Geometry check sheet. Reference: the model listing, model coordinates, mm. A direction names the side the tool comes from. Round coordinates to 2 decimals unless told otherwise and drop trailing zeros. Loops run counter-clockwise (first coordinate to the right, second up) from the corner with the lowest first, then second, coordinate; pieces in that order, holes last. Notation, with made-up numbers: M -37,9.25 L 3,9.25 A17 cw 3,31.25 Z; hole C -12,33 d10. An arc over 180 degrees is marked long. Use one line per item in the form item = value. Start each with the question number.
1. Set-up check for faces 1 (the flat face through (-109, 53, -2)), 2 (the flat face through (-2, 43, -8)), 3 (the conical face through (-171.003, 19.14, -1.875)): record each of +Z, -Z, +X, -X, +Y, -Y from which the full face is reachable in a straight line by a thin tool's end or side.
2. Go/stop test with flat-tipped pins: pin 1 (5 mm diameter, centred on x = -13.38, y = 72.07, fed in from +Z); pin 2 (5 mm diameter, centred on x = -81.5, y = 39.5, fed in from -Z); pin 3 (4 mm diameter, centred on x = -13.38, y = 19.07, fed in from +Z). Record where each tip stops, or that it passes through.
3. Cross-section at D-D (x = -69). Record the boundary of the cut face in (y, z), then the cut area to 3 significant figures.
4. Material ranges on line 1 (Y direction, x = -7.5, z = -4.25); line 2 (X direction, y = 38.5, z = -6); line 3 (Y direction, x = -13, z = -2.5), recorded low to high.
5. Cross-section at B-B (x = -124). Record the boundary of the cut face in (y, z).
6. Draft check along X on faces 4 (the flat face through (-89, 84, -7)), 5 (the flat face through (-91, 43, -4)). Enter one of: pulls with the +X half, pulls with the -X half, needs draft (parallel to the pull), parting line crosses it, or undercut.
7. Cross-section at C-C (z = -7.25). Record the boundary of the cut face in (x, y).
8. Cross-section at A-A (y = 50). Record the boundary of the cut face in (x, z).
```python
from build123d import *

# Parameters (mm, degrees)
F1_DEPTH = 11.5
F0_R     = 1.5
F2_DEPTH = 4
F3_SIZE  = 2
F4_W     = 27.3790522566
F4_H     = 13
F5_DEPTH = 25


# Not quite as in the source:
# - a feature names something its author has since deleted; it is built from what else it names


with BuildPart() as f1:
    # F0 (on Top) → F1 (new body)
    with BuildSketch(Plane.XY):
        Polygon((-180.3790522566, 0), (0, 0), (0, 42), (0, 84), (-180.3790522566, 84), align=None)
        Polygon((-2, 82), (-2, 42), (-2, 2), (-35, 2), (-178.3790522566, 2), (-178.3790522566, 82), (-35, 82), align=None, mode=Mode.SUBTRACT)
    extrude(amount=-F1_DEPTH)

    # F0 (on Top) → F2 (join)
    with BuildSketch(Plane.XY):
        Polygon((-35, 76.0685783849), (-35, 82), (-178.3790522566, 82), (-178.3790522566, 2), (-35, 2), (-35, 15.0685783849), (-63, 15.0685783849), (-173.3790522566, 15.0685783849), (-173.3790522566, 76.0685783849), align=None)
        with BuildLine():
            Line((-35, 63), (-35, 76.0685783849))
            Line((-35, 76.0685783849), (-173.3790522566, 76.0685783849))
            Line((-173.3790522566, 76.0685783849), (-173.3790522566, 15.0685783849))
            Line((-173.3790522566, 15.0685783849), (-63, 15.0685783849))
            Line((-63, 15.0685783849), (-63, 21.5))
            Line((-63, 21.5), (-163, 21.5))
            Line((-163, 21.5), (-163, 62.5))
            Line((-163, 62.5), (-63, 62.5))
            Line((-63, 62.5), (-63, 42))
            Line((-63, 42), (-56, 42))
            ThreePointArc((-56, 42), (-51, 47), (-46, 42))
            Line((-46, 42), (-40, 42))
            ThreePointArc((-40, 42), (-38.5355339059, 45.5355339059), (-35, 47))
            Line((-35, 47), (-35, 53))
            ThreePointArc((-35, 53), (-40, 58), (-35, 63))
        make_face()
        with Locations((-169.3790522566, 19.0685783849)):
            Circle(F0_R, mode=Mode.SUBTRACT)
        with Locations((-169.3790522566, 72.0685783849)):
            Circle(F0_R, mode=Mode.SUBTRACT)
        with BuildLine():
            Line((-14, 42), (-9.3790522566, 42))
            Line((-9.3790522566, 42), (-9.3790522566, 76.0685783849))
            Line((-9.3790522566, 76.0685783849), (-35, 76.0685783849))
            Line((-35, 76.0685783849), (-35, 63))
            ThreePointArc((-35, 63), (-31.4644660941, 61.5355339059), (-30, 58))
            ThreePointArc((-30, 58), (-31.4644660941, 54.4644660941), (-35, 53))
            Line((-35, 53), (-35, 47))
            ThreePointArc((-35, 47), (-31.4644660941, 45.5355339059), (-30, 42))
            Line((-30, 42), (-24, 42))
            ThreePointArc((-24, 42), (-19, 47), (-14, 42))
        make_face()
        with Locations((-13.3790522566, 72.0685783849)):
            Circle(F0_R, mode=Mode.SUBTRACT)
        Polygon((-9.3790522566, 42), (-2, 42), (-2, 82), (-35, 82), (-35, 76.0685783849), (-9.3790522566, 76.0685783849), align=None)
        Polygon((-2, 2), (-2, 42), (-9.3790522566, 42), (-9.3790522566, 15.0685783849), (-35, 15.0685783849), (-35, 2), align=None)
        with BuildLine():
            Line((-9.3790522566, 15.0685783849), (-9.3790522566, 42))
            Line((-9.3790522566, 42), (-14, 42))
            ThreePointArc((-14, 42), (-19, 37), (-24, 42))
            Line((-24, 42), (-30, 42))
            ThreePointArc((-30, 42), (-31.4644660941, 38.4644660941), (-35, 37))
            Line((-35, 37), (-35, 31))
            ThreePointArc((-35, 31), (-31.4644660941, 29.5355339059), (-30, 26))
            ThreePointArc((-30, 26), (-31.4644660941, 22.4644660941), (-35, 21))
            Line((-35, 21), (-35, 15.0685783849))
            Line((-35, 15.0685783849), (-9.3790522566, 15.0685783849))
        make_face()
        with Locations((-13.3790522566, 19.0685783849)):
            Circle(F0_R, mode=Mode.SUBTRACT)
        with BuildLine():
            Line((-63, 15.0685783849), (-35, 15.0685783849))
            Line((-35, 15.0685783849), (-35, 21))
            ThreePointArc((-35, 21), (-40, 26), (-35, 31))
            Line((-35, 31), (-35, 37))
            ThreePointArc((-35, 37), (-38.5355339059, 38.4644660941), (-40, 42))
            Line((-40, 42), (-46, 42))
            ThreePointArc((-46, 42), (-51, 37), (-56, 42))
            Line((-56, 42), (-63, 42))
            Line((-63, 42), (-63, 21.5))
            Line((-63, 21.5), (-63, 15.0685783849))
        make_face()
        with BuildLine():
            Line((-46, 42), (-56, 42))
            ThreePointArc((-56, 42), (-51, 37), (-46, 42))
        make_face()
        with BuildLine():
            ThreePointArc((-46, 42), (-51, 47), (-56, 42))
            Line((-56, 42), (-46, 42))
        make_face()
        with BuildLine():
            ThreePointArc((-35, 37), (-31.4644660941, 38.4644660941), (-30, 42))
            Line((-30, 42), (-35, 42))
            Line((-35, 42), (-35, 37))
        make_face()
        with BuildLine():
            Line((-35, 42), (-30, 42))
            ThreePointArc((-30, 42), (-31.4644660941, 45.5355339059), (-35, 47))
            Line((-35, 47), (-35, 42))
        make_face()
        with BuildLine():
            ThreePointArc((-40, 42), (-38.5355339059, 38.4644660941), (-35, 37))
            Line((-35, 37), (-35, 42))
            Line((-35, 42), (-40, 42))
        make_face()
        with BuildLine():
            Line((-35, 42), (-35, 47))
            ThreePointArc((-35, 47), (-38.5355339059, 45.5355339059), (-40, 42))
            Line((-40, 42), (-35, 42))
        make_face()
        with BuildLine():
            ThreePointArc((-24, 42), (-19, 37), (-14, 42))
            Line((-14, 42), (-24, 42))
        make_face()
        with BuildLine():
            Line((-24, 42), (-14, 42))
            ThreePointArc((-14, 42), (-19, 47), (-24, 42))
        make_face()
        with BuildLine():
            ThreePointArc((-30, 58), (-31.4644660941, 61.5355339059), (-35, 63))
            Line((-35, 63), (-35, 58))
            Line((-35, 58), (-35, 53))
            ThreePointArc((-35, 53), (-31.4644660941, 54.4644660941), (-30, 58))
        make_face()
        with BuildLine():
            Line((-35, 58), (-35, 63))
            ThreePointArc((-35, 63), (-40, 58), (-35, 53))
            Line((-35, 53), (-35, 58))
        make_face()
        with BuildLine():
            Line((-35, 26), (-35, 21))
            ThreePointArc((-35, 21), (-31.4644660941, 22.4644660941), (-30, 26))
            ThreePointArc((-30, 26), (-31.4644660941, 29.5355339059), (-35, 31))
            Line((-35, 31), (-35, 26))
        make_face()
        with BuildLine():
            ThreePointArc((-35, 31), (-40, 26), (-35, 21))
            Line((-35, 21), (-35, 26))
            Line((-35, 26), (-35, 31))
        make_face()
        Polygon((-163, 21.5), (-63, 21.5), (-63, 42), (-63, 62.5), (-163, 62.5), align=None)
    extrude(amount=-F2_DEPTH)

    # F3
    f3_edges = [f1.edges().sort_by_distance(p)[0] for p in [
        (-90.189526, 84, 0),
        (0, 42, 0),
        (-90.189526, 0, 0),
        (-180.379052, 42, 0),
        (-170.879052, 19.068578, 0),
        (-14.879052, 72.068578, 0),
        (-14.879052, 19.068578, 0),
        (-170.879052, 72.068578, 0),
    ]]
    chamfer(f3_edges, length=F3_SIZE)

    # F4 (on face) → F5 (cut)
    with BuildSketch(Plane.XY):
        with Locations((-122.6895261283, 53.5)):
            Rectangle(F4_W, F4_H)
    extrude(amount=-F5_DEPTH, mode=Mode.SUBTRACT)


solid = f1.part
```
Reported:
q1.face_1 = +Z, -Z
q1.face_2 = -Z
q1.face_3 = +Z
q2.pin_1 = -1
q2.pin_2 = -4
q2.pin_3 = -1.5
q3.outline = M 0,-11.5 L 2,-11.5 L 2,-4 L 82,-4 L 82,-11.5 L 84,-11.5 L 84,-2 L 82,0 L 2,0 L 0,-2 Z
q3.area = 362 mm²
q4.line_1 = 0 to 2, 82 to 84
q4.line_2 = -180.38 to -178.38, -2 to 0
q4.line_3 = 0 to 17.62, 20.52 to 70.62, 73.52 to 84
q5.outline = M 0,-11.5 L 2,-11.5 L 2,-4 L 47,-4 L 47,0 L 2,0 L 0,-2 Z; M 60,-4 L 82,-4 L 82,-11.5 L 84,-11.5 L 84,-2 L 82,0 L 60,0 Z
q6.face_4 = needs draft
q6.face_5 = undercut
q7.outline = M -180.38,0 L 0,0 L 0,84 L -180.38,84 Z; hole M -178.38,2 L -2,2 L -2,82 L -178.38,82 Z
q8.outline = M -180.38,-11.5 L -178.38,-11.5 L -178.38,-4 L -136.38,-4 L -136.38,0 L -178.38,0 L -180.38,-2 Z; M -109,-4 L -2,-4 L -2,-11.5 L 0,-11.5 L 0,-2 L -2,0 L -109,0 Z
